Check sheet for the modelled part. Datum: model origin and axes. Units: mm. Face numbers are marked on the shaded views. A direction names the side the tool comes from. Round coordinates to 2 decimals unless told otherwise and drop trailing zeros. Order: outer loops, then holes, each group sorted by start corner. A loop starts at its lowest first (then second) coordinate and runs counter-clockwise, first axis right, second up. Notation, with made-up numbers: (-19.5, 22.5) -> (10.5, 22.5) arc R28 ccw to (10.5, 58.5) -> close; hole circle Ø8 at (58.5, 79.25). An arc over 180 degrees is marked (long way). Use CSV: the item, a comma, the result in double quotes.
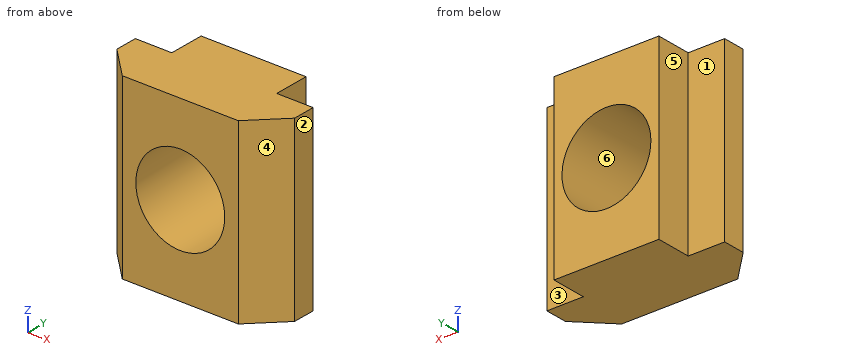
```python
from build123d import *

# Parameters (mm, degrees)
BOSS_EXTRU_1_DEPTH      = 10
ENL_V_MAT_EXTRU_1_REACH = 18.58
ESQUISSE2_R             = 2.5


with BuildPart() as part:
    # Esquisse1 → Boss.-Extru.1 (new body)
    with BuildSketch(Plane.XY):
        Polygon((-10.506087259, -2.086075409), (-3.981368971, -2.086075409), (-2.243728115, -0.348434553), (-2.243728115, 0.913924591), (-4.293728115, 0.913924591), (-4.293728115, 2.913924591), (-10.193728115, 2.913924591), (-10.193728115, 0.913924591), (-12.243728115, 0.913924591), (-12.243728115, -0.348434553), align=None)
    extrude(amount=BOSS_EXTRU_1_DEPTH)

    # Esquisse2 → Enlèv. mat.-Extru.1 (cut, up to next)
    with BuildSketch(Plane(origin=(0, 2.913924591, 0), x_dir=(1, 0, 0), z_dir=(0, 1, 0)), mode=Mode.PRIVATE) as enl_v_mat_extru_1_sk1:
        with Locations(Location((-7.243728115, -5, 0), (0, 0, 270))):
            Circle(ESQUISSE2_R)
    enl_v_mat_extru_1_tool1 = extrude(enl_v_mat_extru_1_sk1.sketch, amount=-ENL_V_MAT_EXTRU_1_REACH, mode=Mode.PRIVATE) & part.part
    add(enl_v_mat_extru_1_tool1.solids().sort_by_distance((-7.243728, 2.913925, 5))[0], mode=Mode.SUBTRACT)


solid = part.part
```
Q1. Go/stop test with flat-tipped pins: pin 1 (1 mm diameter, centred on y = -1.5, z = 8, fed in from -X); pin 2 (0.6 mm diameter, centred on y = 2, z = 7, fed in from -X); pin 3 (2.5 mm diameter, centred on x = -11.5, z = 6.5, fed in from +Y). Record where each tip stops, or that it passes through.
Result sheet:
pin 1,"stops at x = -11.59"
pin 2,"stops at x = -10.19"
pin 3,"stops at y = 0.91"
Q2. Sectioned sample at C-C, the plane z = 1. Enter the section's corners in (x, y), then the cut area to 3 significant figures.
Result sheet:
outline,"(-12.24, -0.35) -> (-10.51, -2.09) -> (-3.98, -2.09) -> (-2.24, -0.35) -> (-2.24, 0.91) -> (-4.29, 0.91) -> (-4.29, 2.91) -> (-10.19, 2.91) -> (-10.19, 0.91) -> (-12.24, 0.91) -> close"
area,"38.8 mm^2"
Q3. Sectioned sample at A-A, the plane z = 5. Enter the section's corners in (x, y), then the cut area to 3 significant figures.
Result sheet:
outline,"(-12.24, -0.35) -> (-10.51, -2.09) -> (-9.74, -2.09) -> (-9.74, 2.91) -> (-10.19, 2.91) -> (-10.19, 0.91) -> (-12.24, 0.91) -> close; (-4.74, -2.09) -> (-3.98, -2.09) -> (-2.24, -0.35) -> (-2.24, 0.91) -> (-4.29, 0.91) -> (-4.29, 2.91) -> (-4.74, 2.91) -> close"
area,"13.8 mm^2"
Q4. Sectioned sample at B-B, the plane x = -9. Enter the section's corners in (y, z).
Result sheet:
outline,"(-2.09, 0) -> (2.91, 0) -> (2.91, 3.22) -> (-2.09, 3.22) -> close; (-2.09, 6.78) -> (2.91, 6.78) -> (2.91, 10) -> (-2.09, 10) -> close"
Q5. Scan lines: L1, parallel to X at y = 1.7, z = 5; L2, parallel to Z at x = -7.25, y = -1.35; L3, parallel to X at y = 2.3, z = 1.25. Record each from-to range of solid material in increasing order.
Result sheet:
L1,"x = -10.19 to -9.74, -4.74 to -4.29"
L2,"z = 0 to 2.5, 7.5 to 10"
L3,"x = -10.19 to -4.29"
Q6. Mould release check, pull along X, two halves, no side actions. Record for the marked faces 4, 5 and 6: pulls with the +X half, pulls with the -X half, needs draft (parallel to the pull), parting line crosses it, or undercut.
Result sheet:
face 4,"pulls with the +X half"
face 5,"pulls with the -X half"
face 6,"undercut"
Q7. Sectioned sample at D-D, the plane y = 0.5. Enter the section's corners in (x, z).
Result sheet:
outline,"(-12.24, 0) -> (-2.24, 0) -> (-2.24, 10) -> (-12.24, 10) -> close; hole circle Ø5 at (-7.24, 5)"
Q8. Access from +Z, -Z, +X, -X, +Y, -Y to the whole of each face (thin tool, end or side, straight path). Record for the marked faces 1, 2 and 3.
Result sheet:
face 1,"+Z, -Z, -X, +Y"
face 2,"+Z, -Z, +X, +Y, -Y"
face 3,"+Z, -Z, +X, +Y"
